Answer from the drawing. Dimensions are ordinates in mm from the lowest x, y and z of the part. Coordinates: 2 decimals unless noted, no trailing zeros. Order: outer loops, then holes, each group sorted by start corner. A loop starts at its lowest first (then second) coordinate and runs counter-clockwise, first axis right, second up. Notation, with made-up numbers: (-12, 43.25) -> (12, 43.25) arc R7 cw to (12, 55.25) -> close; hole circle Ø2 at (70, 82.25). An arc over 180 degrees is marked (long way). Use CSV: the item, a comma, the result in double quotes.
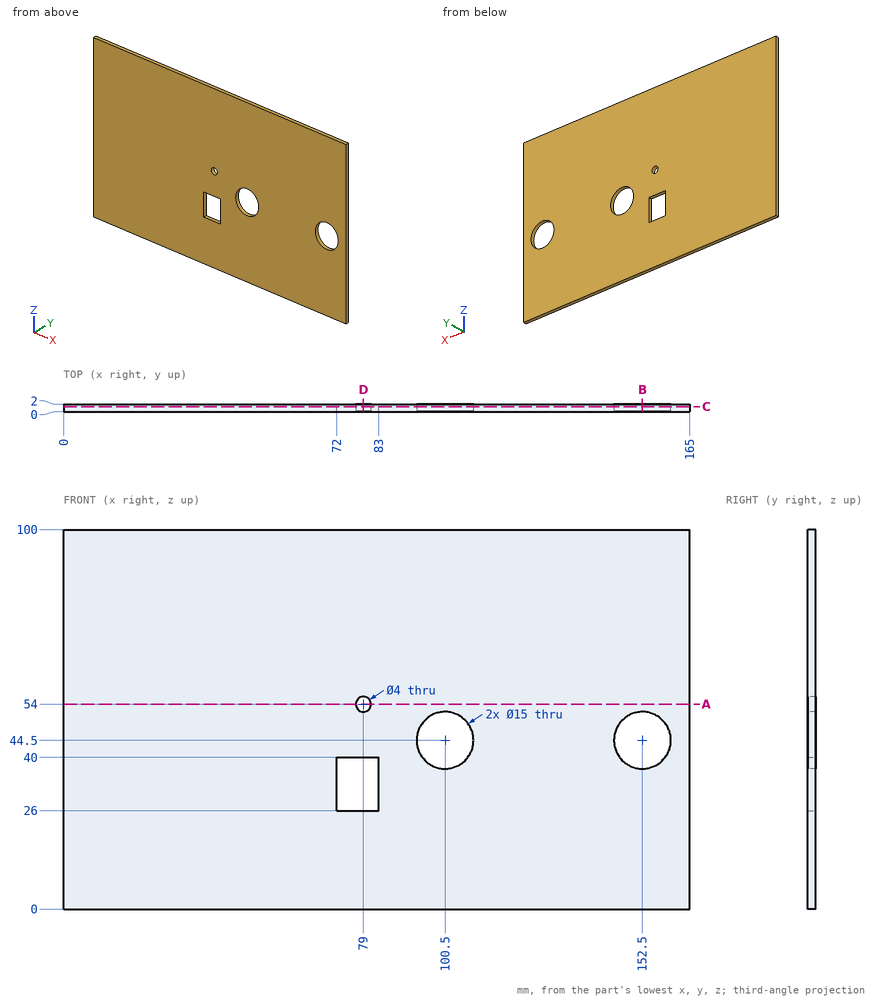
Item 1: Find section C-C, the plane y = 1.3. Give the vertices of the cut face in (x, z).
Return value:
outline,"(0, 0) -> (165, 0) -> (165, 100) -> (0, 100) -> close; hole (72, 26) -> (83, 26) -> (83, 40) -> (72, 40) -> close; hole circle Ø4 at (79, 54); hole circle Ø15 at (100.5, 44.5); hole circle Ø15 at (152.5, 44.5)"
Item 2: Find section B-B, the plane x = 152.5. Give the vertices of the cut face in (y, z).
Return value:
outline,"(0, 0) -> (2, 0) -> (2, 37) -> (0, 37) -> close; (0, 52) -> (2, 52) -> (2, 100) -> (0, 100) -> close"
Item 3: Straight lines are drawn through the part: line 1 along Z through (x, y) = (79, 0.4); line 2 along Z through (x, y) = (100.5, 1.1); line 3 along X through (y, z) = (0.1, 46.5). For each, find the intervals that lie inside material, in ascending order.
Return value:
line 1,"z = 0 to 26, 40 to 52, 56 to 100"
line 2,"z = 0 to 37, 52 to 100"
line 3,"x = 0 to 93.27, 107.73 to 145.27, 159.73 to 165"
Item 4: Find section A-A, the plane z = 54. Give the vertices of the cut face in (x, y), then the cut area to 3 significant figures.
Return value:
outline,"(0, 0) -> (77, 0) -> (77, 2) -> (0, 2) -> close; (81, 0) -> (165, 0) -> (165, 2) -> (81, 2) -> close"
area,"322 mm^2"
Item 5: Find section D-D, the plane x = 79. Give the vertices of the cut face in (y, z).
Return value:
outline,"(0, 0) -> (2, 0) -> (2, 26) -> (0, 26) -> close; (0, 40) -> (2, 40) -> (2, 52) -> (0, 52) -> close; (0, 56) -> (2, 56) -> (2, 100) -> (0, 100) -> close"
